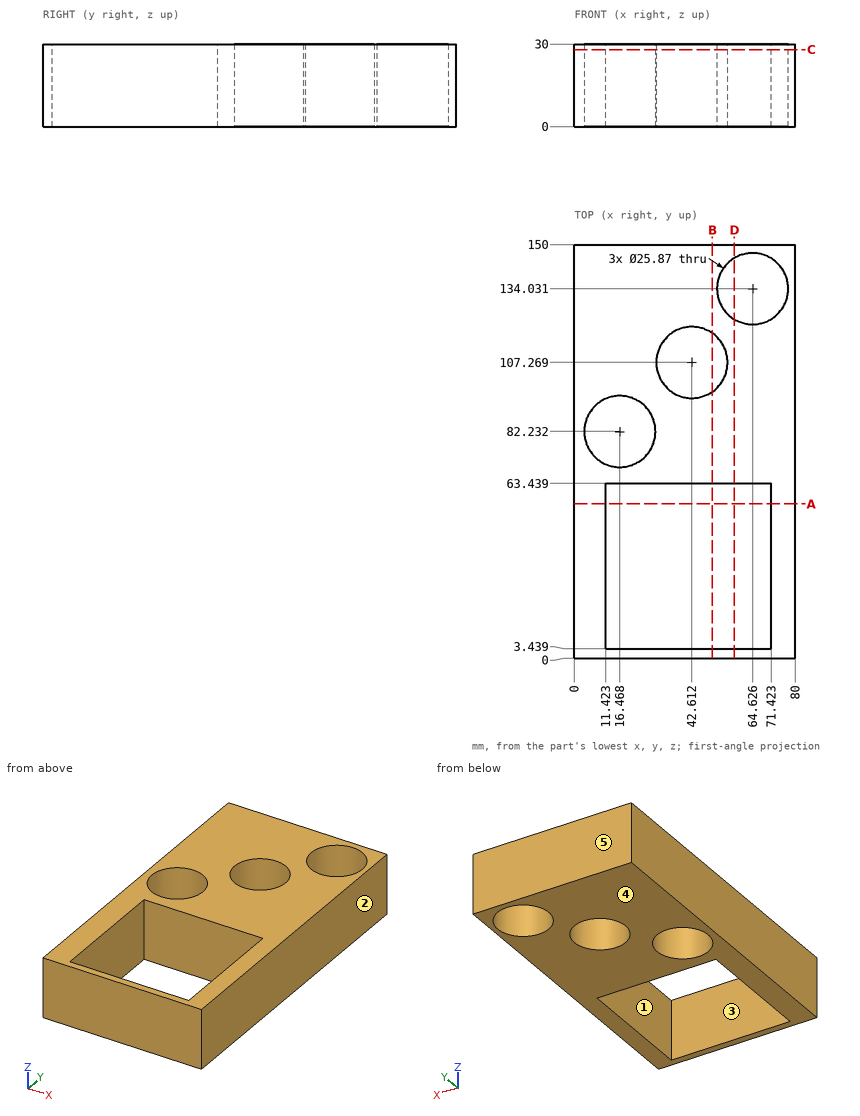
Design review of the part shown in the three views and the two pictorial views. Dimensions are in mm from the part's minimum x, y and z. A direction names the side the tool comes from. Coordinates: 2 decimals unless noted, no trailing zeros. Order: outer loops, then holes, each group sorted by start corner. A loop starts at its lowest first (then second) coordinate and runs counter-clockwise, first axis right, second up.
1) Take a section at C-C, the plane z = 28. Give the boundary of the cut face in (x, y) (1 decimal), and give its area (3 significant figures).
2) Clearance check with a flat-ended pin moving along its axis: pin 1 (23.5 mm diameter, centred on x = 64.63, y = 134.03, fed in from +Z). State where the tip first meets the part, or that it passes through.
3) Mouldability with a two-part tool opening along Y and no side actions: class the marked faces 3, 4 and 5 as +Y half, -Y half, draft (parallel to the pull), parting line (faces both ways), or undercut.
4) Wall thickness on line 1 along X through (y, z) = (6, 6.25); line 2 along Y through (x, z) = (18, 15.25) (1 decimal); line 3 along Y through (x, z) = (66, 24): over which ranges is each line inside the solid? List them lowest first.
5) Take a section at D-D, the plane x = 58. Give the boundary of the cut face in (y, z).
6) Take a section at B-B, the plane x = 50. Give the boundary of the cut face in (y, z), and give its area (3 significant figures).
7) Take a section at A-A, the plane y = 56. Give the boundary of the cut face in (x, z).
8) For the marked faces 1 and 2, list the 3-axis set-ups (+Z, -Z, +X, -X, +Y, -Y) from which the entire face can be reached by the end or side of a thin tool; tool diameter is ignored.
Returned:
1. outline: (0, 0) - (80, 0) - (80, 150) - (0, 150) - close; hole circle Ø25.9 at (16.5, 82.2); hole (11.4, 3.4) - (71.4, 3.4) - (71.4, 63.4) - (11.4, 63.4) - close; hole circle Ø25.9 at (42.6, 107.3); hole circle Ø25.9 at (64.6, 134)
1. area: 6,820 mm2
2. pin 1: passes through
3. face 3: undercut
3. face 4: draft
3. face 5: +Y half
4. line 1: x = 0 to 11.42, 71.42 to 80
4. line 2: y = 0 to 3.4, 63.4 to 69.4, 95.1 to 150
4. line 3: y = 0 to 3.44, 63.44 to 121.17, 146.89 to 150
5. outline: (0, 0) - (3.44, 0) - (3.44, 30) - (0, 30) - close; (63.44, 0) - (122.92, 0) - (122.92, 30) - (63.44, 30) - close; (145.14, 0) - (150, 0) - (150, 30) - (145.14, 30) - close
6. outline: (0, 0) - (3.44, 0) - (3.44, 30) - (0, 30) - close; (63.44, 0) - (96.65, 0) - (96.65, 30) - (63.44, 30) - close; (117.89, 0) - (150, 0) - (150, 30) - (117.89, 30) - close
6. area: 2,060 mm2
7. outline: (0, 0) - (11.42, 0) - (11.42, 30) - (0, 30) - close; (71.42, 0) - (80, 0) - (80, 30) - (71.42, 30) - close
8. face 1: +Z, -Z
8. face 2: +Z, -Z, +X, +Y, -Y
